Design review of the part built by this model. Coordinates are the model's own, in mm. Face numbers are marked on the shaded views. A direction names the side the tool comes from. Round coordinates to 2 decimals unless told otherwise and drop trailing zeros. Write each loop counter-clockwise with the first axis right and the second up, starting at its lowest first coordinate (ties: lowest second). Pieces come first, ordered by that corner, then holes. Notation, with made-up numbers: (45, 25.5) -> (60, 25.5) arc R18 ccw to (60, 45.5) -> close; hole circle Ø10 at (61, 0). An arc over 180 degrees is marked (long way). Write item = value, one per line. Start each with the question number.
Item 1: Mouldability with a two-part tool opening along Z and no side actions: class the marked faces 1, 2 and 3 as released by +Z, released by -Z, zero draft, split by the parting line, or undercut.
Item 2: Add section A-A, the plane z = 0. State the section outline as (x, y) points.
Item 3: Add section B-B, the plane x = -7.5. State the section outline as (y, z) points.
Item 4: Machinability: for the marked faces 4, 5 and 6, which of the approach directions +Z, -Z, +X, -X, +Y, -Y give a long, thin tool a straight path to every point of the face, cutting with its end or side? Answer none if there is none.
Item 5: To check wall thickness, follow L1, parallel to Z at x = 0, y = 10; L2, parallel to X at y = 30, z = 26; L3, parallel to Z at x = 0, y = 5. State the ranges of each line that lie inside material, in increasing order.
Item 6: For pin 1 Ø10 at (x, z) = (-3, 26) entering from -Y; pin 2 Ø3 at (x, z) = (0, 26) entering from +Y, all flat-tipped, find the tip position at first contact; note any pin that passes through.
Item 7: Add section C-C, the plane y = 13.5. State the section outline as (x, z) points.
Item 8: Add section D-D, the plane z = 20.5. State the section outline as (x, y) points.
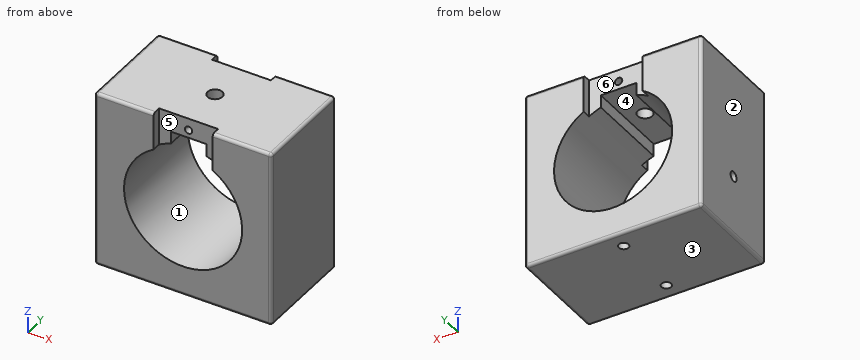
from build123d import *

# Parameters (mm, degrees)
ESQUISSE1_W             = 60
ESQUISSE1_H             = 60
ESQUISSE1_R             = 20
BOSS_EXTRU_1_DEPTH      = 35
CONG_1_R                = 1
TROU_TARAUD_M61_REACH   = 77.664
TROU_TARAUD_M61_BORE_R  = 2.5
TROU_TARAUD_M41_D       = 3.3
TROU_TARAUD_M41_DEPTH   = 7.5
TROU_TARAUD_M41_TIP     = 0.991420021
TROU_TARAUD_M42_D       = 3.3
TROU_TARAUD_M42_DEPTH   = 10.5
TROU_TARAUD_M42_TIP     = 0.991420021
ENL_V_MAT_EXTRU_1_REACH = 57
ENL_V_MAT_EXTRU_2_DEPTH = 3


with BuildPart() as part:
    # Esquisse1 → Boss.-Extru.1 (new body)
    with BuildSketch(Plane(origin=(0, 0, 0), x_dir=(1, 0, 0), z_dir=(0, 1, 0))):
        Rectangle(ESQUISSE1_W, ESQUISSE1_H)
        with Locations(Location((0, 0, 0), (0, 0, 270))):
            Circle(ESQUISSE1_R, mode=Mode.SUBTRACT)
    extrude(amount=BOSS_EXTRU_1_DEPTH)

    # Congé1
    cong_1_edges = [part.edges().sort_by_distance(p)[0] for p in [
        (30, 35, 0),
        (0, 35, -30),
        (-30, 35, 0),
        (0, 0, -30),
        (30, 0, 0),
        (0, 0, 30),
        (-30, 0, 0),
        (0, 35, 30),
        (-30, 17.5, -30),
        (30, 17.5, -30),
        (30, 17.5, 30),
        (-30, 17.5, 30),
    ]]
    fillet(cong_1_edges, radius=CONG_1_R)

    # Trou taraudé M61 bore → Trou taraudé M61 (cut, up to next)
    with BuildSketch(Plane.XY.offset(30), mode=Mode.PRIVATE) as trou_taraud_m61_sk1:
        with Locations((0, 17.5)):
            Circle(TROU_TARAUD_M61_BORE_R)
    trou_taraud_m61_tool1 = extrude(trou_taraud_m61_sk1.sketch, amount=-TROU_TARAUD_M61_REACH, mode=Mode.PRIVATE) & part.part
    add(trou_taraud_m61_tool1.solids().sort_by_distance((0, 17.5, 30))[0], mode=Mode.SUBTRACT)

    # Trou taraudé M41
    with Locations(Plane(origin=(0, 0, -30), x_dir=(-1, 0, 0), z_dir=(0, 0, -1))):
        with Locations((0, 29.2), (0, 5.8)):
            Hole(TROU_TARAUD_M41_D / 2, depth=TROU_TARAUD_M41_DEPTH)
            with Locations((0, 0, -(TROU_TARAUD_M41_DEPTH + TROU_TARAUD_M41_TIP / 2))):  # 118° drill point
                Cone(0, TROU_TARAUD_M41_D / 2, TROU_TARAUD_M41_TIP, mode=Mode.SUBTRACT)

    # Trou taraudé M42
    with Locations(Plane.ZY.offset(30)):
        with Locations((-9.666666667, 17.5)):
            Hole(TROU_TARAUD_M42_D / 2, depth=TROU_TARAUD_M42_DEPTH)
            with Locations((0, 0, -(TROU_TARAUD_M42_DEPTH + TROU_TARAUD_M42_TIP / 2))):  # 118° drill point
                Cone(0, TROU_TARAUD_M42_D / 2, TROU_TARAUD_M42_TIP, mode=Mode.SUBTRACT)

    # Esquisse10 → Enlèv. mat.-Extru.1 (cut, up to next)
    with BuildSketch(Plane.XZ, mode=Mode.PRIVATE) as enl_v_mat_extru_1_sk1:
        with BuildLine():
            Line((6, 23.3), (6, 19.078784028))
            ThreePointArc((6, 19.078784028), (0, 20), (-6, 19.078784028))
            Line((-6, 19.078784028), (-6, 23.3))
            Line((-6, 23.3), (6, 23.3))
        make_face()
    enl_v_mat_extru_1_tool1 = extrude(enl_v_mat_extru_1_sk1.sketch, amount=-ENL_V_MAT_EXTRU_1_REACH, mode=Mode.PRIVATE) & part.part
    add(enl_v_mat_extru_1_tool1.solids().sort_by_distance((0, 0, 21.487514))[0], mode=Mode.SUBTRACT)

    # Esquisse11 → Enlèv. mat.-Extru.2 (cut)
    with BuildSketch(Plane.XZ):
        with BuildLine():
            Line((-10, 30), (-10, 17.320508076))
            ThreePointArc((-10, 17.320508076), (0, 20), (10, 17.320508076))
            Line((10, 17.320508076), (10, 30))
            Line((10, 30), (-10, 30))
        make_face()
    enl_v_mat_extru_2 = extrude(amount=-ENL_V_MAT_EXTRU_2_DEPTH, mode=Mode.SUBTRACT)

    # Esquisse13 → Trou taraudé M31 (revolve, cut)
    with BuildSketch(Plane(origin=(0, 3, 26), x_dir=(0, 0, -1), z_dir=(1, 0, 0))):
        Polygon((0, 0), (0, 9.251075774), (1.25, 8.5), (1.25, 0), align=None)
    trou_taraud_m31 = revolve(axis=Axis((0, -3.35, 26), (0, 1, 0)), mode=Mode.SUBTRACT)

    # Symétrie1: Enlèv. mat.-Extru.2, Trou taraudé M31 across plane
    add(enl_v_mat_extru_2.mirror(Plane(origin=(0, 17.5, 0), x_dir=(0, 0, 1), z_dir=(0, -1, 0))), mode=Mode.SUBTRACT)
    add(trou_taraud_m31.mirror(Plane(origin=(0, 17.5, 0), x_dir=(0, 0, 1), z_dir=(0, -1, 0))), mode=Mode.SUBTRACT)


solid = part.part
Result set:
q1.face_1 = undercut
q1.face_2 = zero draft
q1.face_3 = released by -Z
q2.outline = (-30, 1) arc R1 ccw to (-29, 0) -> (-20, 0) -> (-20, 35) -> (-29, 35) arc R1 ccw to (-30, 34) -> close; (20, 0) -> (29, 0) arc R1 ccw to (30, 1) -> (30, 34) arc R1 ccw to (29, 35) -> (20, 35) -> close
q3.outline = (0, -29) arc R1 ccw to (1, -30) -> (34, -30) arc R1 ccw to (35, -29) -> (35, -18.54) -> (0, -18.54) -> close; (3, 18.54) -> (32, 18.54) -> (32, 30) -> (3, 30) -> close
q4.face_4 = +Y, -Y
q4.face_5 = +Z, -Y
q4.face_6 = +Z, +Y
q5.L1 = -30 to -20, 23.3 to 24.75, 27.25 to 30
q5.L2 = -30 to -1.25, 1.25 to 30
q5.L3 = -21.99 to -20, 23.3 to 24.75, 27.25 to 30
q6.pin_1 = 3
q6.pin_2 = 32
q7.outline = (-30, -29) arc R1 ccw to (-29, -30) -> (29, -30) arc R1 ccw to (30, -29) -> (30, 29) arc R1 ccw to (29, 30) -> (-29, 30) arc R1 ccw to (-30, 29) -> close; hole (-6, 19.08) arc R20 ccw (long way) to (6, 19.08) -> (6, 23.3) -> (-6, 23.3) -> close
q8.outline = (-30, 1) arc R1 ccw to (-29, 0) -> (-10, 0) -> (-10, 3) -> (-6, 3) -> (-6, 32) -> (-10, 32) -> (-10, 35) -> (-29, 35) arc R1 ccw to (-30, 34) -> close; (6, 3) -> (10, 3) -> (10, 0) -> (29, 0) arc R1 ccw to (30, 1) -> (30, 34) arc R1 ccw to (29, 35) -> (10, 35) -> (10, 32) -> (6, 32) -> close
